from build123d import *

# Parameters (mm, degrees)
SKETCH1_W                 = 54.61
SKETCH1_H                 = 50.8
BOSS_EXTRUDE1_DEPTH       = 6.35
F_4_40_TAPPED_HOLE1_D     = 2.2606
F_4_40_TAPPED_HOLE1_DEPTH = 6.35
F_4_CLEARANCE_HOLE1_D     = 3.2639
F_4_CLEARANCE_HOLE1_DEPTH = 6.35


with BuildPart() as part:
    # Sketch1 → Boss-Extrude1 (new body)
    with BuildSketch(Plane(origin=(0, 0, 0), x_dir=(1, 0, 0), z_dir=(0, 1, 0))):
        Rectangle(SKETCH1_W, SKETCH1_H)
    extrude(amount=BOSS_EXTRUDE1_DEPTH)

    # #4-40 Tapped Hole1
    with Locations(Plane(origin=(0, 6.35, 0), x_dir=(1, 0, 0), z_dir=(0, 1, 0))):
        with Locations((-25, 15), (8e-07, 15), (25.0000016, 15), (8e-07, -14.9999908), (25.0000016, -14.9999908), (-25, -14.9999908)):
            Hole(F_4_40_TAPPED_HOLE1_D / 2, depth=F_4_40_TAPPED_HOLE1_DEPTH)

    # #4 Clearance Hole1
    with Locations(Plane(origin=(0, 6.35, 0), x_dir=(1, 0, 0), z_dir=(0, 1, 0))):
        with Locations((-25, 22.86), (0, 22.86), (25, 22.86), (0, -22.86), (25, -22.86), (-25, -22.86)):
            Hole(F_4_CLEARANCE_HOLE1_D / 2, depth=F_4_CLEARANCE_HOLE1_DEPTH)


solid = part.part
Work out the finished part from the listing and answer in its coordinate system (mm). Round coordinates to 2 decimals unless told otherwise and drop trailing zeros. Write each loop counter-clockwise with the first axis right and the second up, starting at its lowest first coordinate (ties: lowest second). Pieces come first, ordered by that corner, then holes.
1) A cutting plane is placed at C-C (y = 2.75). Give the number of separate pieces and of enclosed holes in the cut face, plus the area to 3 significant figures.
2) A cutting plane is placed at D-D (z = -15). Give the vertices of the cut face in (x, y) (3 decimals).
3) Straight lines are drawn through the part: line 1 (Z direction, x = 0, y = 4.75); line 2 (X direction, y = 1.75, z = 15) (3 decimals); line 3 (X direction, y = 1.5, z = -22.86) (3 decimals). For each, find the intervals that lie inside material, in ascending order.
4) A cutting plane is placed at A-A (z = 22.86). Give the vertices of the cut face in (x, y) (3 decimals), plus the area to 3 significant figures.
5) A cutting plane is placed at B-B (x = 0). Give the vertices of the cut face in (y, z).
6) The mould has two halves that part along Z. Classify faces 1 (the flat face through (0, 6.35, 0)), 2 (the flat face through (0, 3, 25.4)), 3 (the cylindrical face through (0.354, 3.131, 24.453)): pulls with the +Z half, pulls with the -Z half, needs draft (parallel to the pull), parting line crosses it, or undercut.
Completed:
1. separate pieces: 1
1. enclosed holes: 12
1. area: 2,700 mm2
2. outline: (-27.305, 0) - (-26.13, 0) - (-26.13, 6.35) - (-27.305, 6.35) - close; (-23.87, 0) - (-1.13, 0) - (-1.13, 6.35) - (-23.87, 6.35) - close; (1.13, 0) - (23.87, 0) - (23.87, 6.35) - (1.13, 6.35) - close; (26.13, 0) - (27.305, 0) - (27.305, 6.35) - (26.13, 6.35) - close
3. line 1: z = -25.4 to -24.49, -21.23 to -16.13, -13.87 to 13.87, 16.13 to 21.23, 24.49 to 25.4
3. line 2: x = -27.305 to -26.13, -23.87 to -1.13, 1.13 to 23.87, 26.13 to 27.305
3. line 3: x = -27.305 to -26.632, -23.368 to -1.632, 1.632 to 23.368, 26.632 to 27.305
4. outline: (-27.305, 0) - (-26.632, 0) - (-26.632, 6.35) - (-27.305, 6.35) - close; (-23.368, 0) - (-1.632, 0) - (-1.632, 6.35) - (-23.368, 6.35) - close; (1.632, 0) - (23.368, 0) - (23.368, 6.35) - (1.632, 6.35) - close; (26.632, 0) - (27.305, 0) - (27.305, 6.35) - (26.632, 6.35) - close
4. area: 285 mm2
5. outline: (0, -25.4) - (6.35, -25.4) - (6.35, -24.49) - (0, -24.49) - close; (0, -21.23) - (6.35, -21.23) - (6.35, -16.13) - (0, -16.13) - close; (0, -13.87) - (6.35, -13.87) - (6.35, 13.87) - (0, 13.87) - close; (0, 16.13) - (6.35, 16.13) - (6.35, 21.23) - (0, 21.23) - close; (0, 24.49) - (6.35, 24.49) - (6.35, 25.4) - (0, 25.4) - close
6. face 1: needs draft
6. face 2: pulls with the +Z half
6. face 3: undercut
